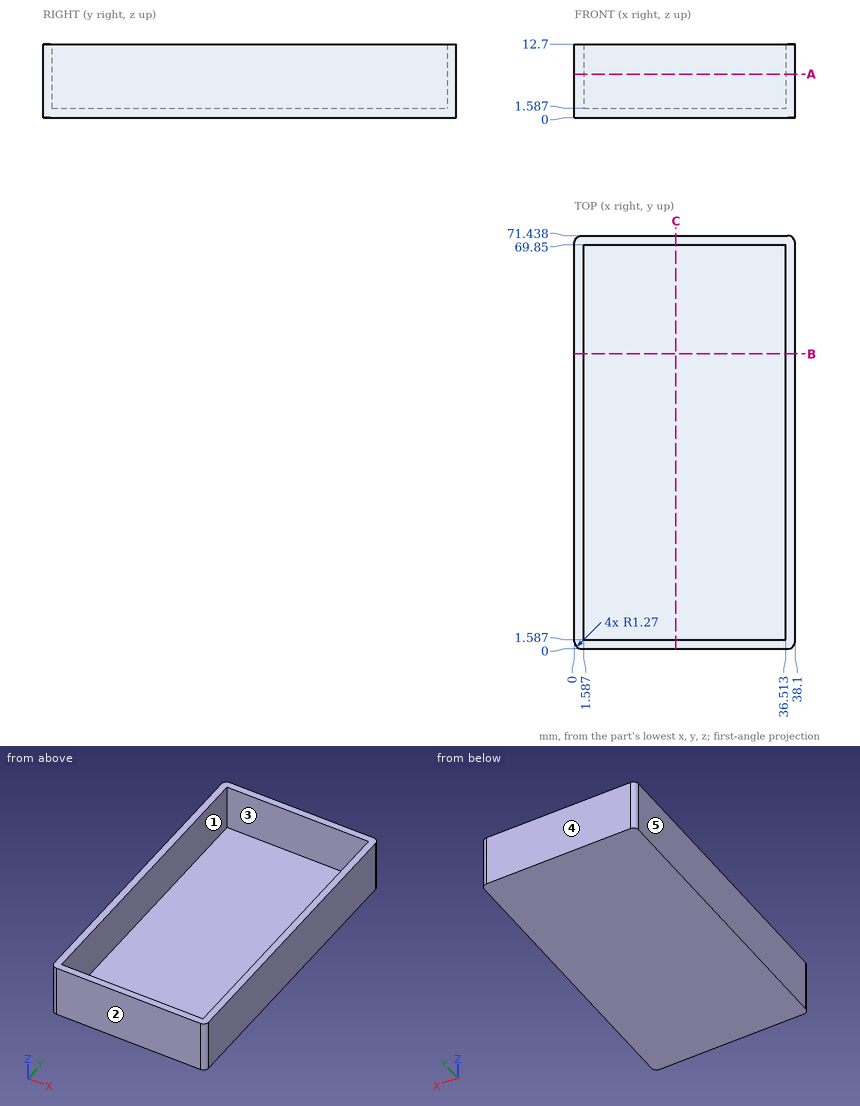
Verification items for this drawing (mm, ordinates from the low corner). A direction names the side the tool comes from. Give positions to 0.01 mm unless a question says otherwise; leave off trailing zeros. Write each loop counter-clockwise with the first axis right and the second up, starting at its lowest first coordinate (ties: lowest second). Pieces come first, ordered by that corner, then holes.
1) Gauge pin test, flat ends, axial feed: pin 1 (10.5 mm diameter, centred on x = 19.5, y = 29.5, fed in from +Z); pin 2 (6 mm diameter, centred on x = 24.5, z = 8.5, fed in from -Y). Record the tip position at first contact, or that the pin passes through.
2) Section check A-A, the plane z = 7.5. Record the boundary of the cut face in (x, y).
3) Material ranges on L1, parallel to X at y = 21.5, z = 6; L2, parallel to Y at x = 22, z = 7; L3, parallel to Z at x = 29, y = 60, recorded low to high.
4) Access from +Z, -Z, +X, -X, +Y, -Y to the whole of each face (thin tool, end or side, straight path). Record for the marked faces 1 and 2.
5) Section check B-B, the plane y = 51. Record the boundary of the cut face in (x, z).
6) Section check C-C, the plane x = 17.5. Record the boundary of the cut face in (y, z).
7) Release check for a two-part mould opening along X. For the marked faces 3, 4 and 5 record: pulls with the +X half, pulls with the -X half, needs draft (parallel to the pull), parting line crosses it, or undercut.
Computed:
1. pin 1: stops at z = 1.59
1. pin 2: stops at y = 0
2. outline: (0, 1.27) arc R1.27 ccw to (1.27, 0) - (36.83, 0) arc R1.27 ccw to (38.1, 1.27) - (38.1, 70.17) arc R1.27 ccw to (36.83, 71.44) - (1.27, 71.44) arc R1.27 ccw to (0, 70.17) - close; hole (1.59, 1.59) - (36.51, 1.59) - (36.51, 69.85) - (1.59, 69.85) - close
3. L1: x = 0 to 1.59, 36.51 to 38.1
3. L2: y = 0 to 1.59, 69.85 to 71.44
3. L3: z = 0 to 1.59
4. face 1: +Z
4. face 2: +Z, -Z, +X, -X, -Y
5. outline: (0, 0) - (38.1, 0) - (38.1, 12.7) - (36.51, 12.7) - (36.51, 1.59) - (1.59, 1.59) - (1.59, 12.7) - (0, 12.7) - close
6. outline: (0, 0) - (71.44, 0) - (71.44, 12.7) - (69.85, 12.7) - (69.85, 1.59) - (1.59, 1.59) - (1.59, 12.7) - (0, 12.7) - close
7. face 3: undercut
7. face 4: needs draft
7. face 5: pulls with the -X half
